```python
from build123d import *

# Parameters (mm, degrees)
SKETCH_1_W          = 60
SKETCH_1_H          = 16
EXTRUDE_1_DEPTH     = 3
SKETCH_2_W          = 60
SKETCH_2_H          = 4
EXTRUDE_2_DEPTH     = 100
SKETCH_3_W          = 5
SKETCH_3_H          = 3
EXTRUDE_3_DEPTH     = 30
CUT_EXTRUDE_2_DEPTH = 12
FILLET_2_R          = 5
SKETCH_6_W          = 5
SKETCH_6_H          = 16
CUT_EXTRUDE_3_DEPTH = 12


with BuildPart() as part:
    # 草图1 → 凸台-拉伸1 (new body)
    with BuildSketch(Plane.XY):
        with Locations((7.850953206, 0.370883882)):
            Rectangle(SKETCH_1_W, SKETCH_1_H)
    extrude(amount=EXTRUDE_1_DEPTH)

    # 草图2 → 凸台-拉伸2 (add)
    with BuildSketch(Plane.XY.offset(3)):
        with Locations((7.850953206, -0.129116118)):
            Rectangle(SKETCH_2_W, SKETCH_2_H)
    extrude(amount=EXTRUDE_2_DEPTH)

    # 草图3 → 凸台-拉伸3 (add)
    with BuildSketch(Plane.XZ.offset(2.129116118)):
        with Locations((-4.649046794, 101.5)):
            Rectangle(SKETCH_3_W, SKETCH_3_H)
        with Locations((20.350953206, 101.5)):
            Rectangle(SKETCH_3_W, SKETCH_3_H)
    extrude(amount=EXTRUDE_3_DEPTH)

    # 草图4 → 切除-拉伸2 (cut)
    with BuildSketch(Plane.XZ.offset(2.129116118)):
        Polygon((-7.149046794, 103), (-22.149046794, 103), (-22.149046794, 3), (-7.149046794, 3), (-7.149046794, 100), align=None)
        Polygon((-2.149046794, 42.479838541), (-2.149046794, 3), (17.850953206, 3), (17.850953206, 10.460890497), (16.154674687, 13.176543186), align=None)
        Polygon((17.850953206, 71.715630146), (17.850953206, 18.011289252), (0.231428364, 46.219221776), align=None)
        Polygon((15.355477041, 75.140410003), (-2.149046794, 49.810414331), (-2.149046794, 96.816642788), align=None)
        Polygon((22.850953206, 100), (22.850953206, 3), (37.850953206, 3), (37.850953206, 103), (22.850953206, 103), align=None)
        Polygon((17.850953206, 100), (17.850953206, 78.416921986), (0.421656, 100), align=None)
    extrude(amount=-CUT_EXTRUDE_2_DEPTH, mode=Mode.SUBTRACT)

    # 圆角2
    fillet_2_edges = [part.edges().sort_by_distance(p)[0] for p in [
        (17.850953206, -0.129116118, 3),
        (-2.149046794, -0.129116118, 3),
        (22.850953206, -0.129116118, 3),
        (20.350953206, 1.870883882, 3),
        (-4.649046794, 1.870883882, 3),
        (-4.649046794, -2.129116118, 3),
        (20.350953206, -2.129116118, 3),
        (-7.149046794, -0.129116118, 3),
    ]]
    fillet(fillet_2_edges, radius=FILLET_2_R)

    # 草图6 → 切除-拉伸3 (cut)
    with BuildSketch(Plane.XY.offset(3)):
        with Locations((-19.649046794, 0.370883882)):
            Rectangle(SKETCH_6_W, SKETCH_6_H)
        with Locations((35.350953206, 0.370883882)):
            Rectangle(SKETCH_6_W, SKETCH_6_H)
    extrude(amount=-CUT_EXTRUDE_3_DEPTH, mode=Mode.SUBTRACT)


solid = part.part
```
Source: CAD feature listing. Evaluate the final solid. Frame: model axes, mm. A direction names the side the tool comes from. Give positions to 0.01 mm unless a question says otherwise; leave off trailing zeros. Loops run counter-clockwise (first coordinate to the right, second up) from the corner with the lowest first, then second, coordinate; pieces in that order, holes last. Notation, with made-up numbers: M 47,16 L 52,16 A35 ccw 52,51 Z; hole C 3.25,17 d3. An arc over 180 degrees is marked long. Put each result on its own line as item: value.
Q1. Section D-D (x = 21). Return the cut outline in (y, z), and give its area (3 significant figures).
Response values:
outline: M -32.13,100 L -2.13,100 L -2.13,8 A5 cw -7.13,3 L -7.63,3 L -7.63,0 L 8.37,0 L 8.37,3 L 6.87,3 A5 cw 1.87,8 L 1.87,103 L -32.13,103 Z
area: 549 mm²
Q2. Line query: probe 1 along Y at (x, z) = (19.5, 59.5); probe 2 along X at (y, z) = (-2, 66.5); probe 3 along Z at (x, y) = (-6, -15.5). Output: solid intervals per line, ascending. Write a range as [from, to].
Response values:
probe 1: y = [-2.13, 1.87]
probe 2: x = [-7.15, -2.15], [9.38, 14.25], [17.85, 22.85]
probe 3: z = [100, 103]
Q3. Section A-A (y = -26). Return the cut outline in (x, z), and give its area (3 significant figures).
Response values:
outline: M -7.15,100 L -2.15,100 L -2.15,103 L -7.15,103 Z; M 17.85,100 L 22.85,100 L 22.85,103 L 17.85,103 Z
area: 30.0 mm²
Q4. Mould query, pull axis Z, two halves, no side actions, for faces 1 (the flat face through (-17.149, 0, 2)), 2 (the flat face through (-2.4, -11.1, 103)), 3 (the cylindrical face through (15.67, -0.03, 3.87)). Classes: released by +Z, released by -Z, zero draft, split by the parting line, or undercut.
Response values:
face 1: zero draft
face 2: released by +Z
face 3: undercut
Q5. Section B-B (y = 0). Return the cut outline in (x, z), and give its area (3 significant figures).
Response values:
outline: M -17.15,0 L 32.85,0 L 32.85,3 L 27.85,3 A5 cw 22.85,8 L 22.85,103 L -7.15,103 L -7.15,8 A5 cw -12.15,3 L -17.15,3 Z; hole M -2.15,8 A5 ccw 2.85,3 L 12.85,3 A5 ccw 17.85,8 L 17.85,10.46 L -2.15,42.48 Z; hole M -2.15,49.81 L 15.36,75.14 L -2.15,96.82 Z; hole M 0.23,46.22 L 17.85,18.01 L 17.85,71.72 Z; hole M 0.42,100 L 17.85,78.42 L 17.85,100 Z
area: 1,630 mm²
Q6. Section C-C (y = -5.5). Return the cut outline in (x, z), and give its area (3 significant figures).
Response values:
outline: M -17.15,0 L 32.85,0 L 32.85,3 L 27.85,3 A5 cw 26.22,3.27 L 14.48,3.27 A5 cw 12.85,3 L 2.85,3 A5 cw 1.22,3.27 L -10.52,3.27 A5 cw -12.15,3 L -17.15,3 Z; M -7.15,100 L -2.15,100 L -2.15,103 L -7.15,103 Z; M 17.85,100 L 22.85,100 L 22.85,103 L 17.85,103 Z
area: 187 mm²
Q7. Reachability of faces 4 (the flat face through (17.851, -17, 101)), 5 (the flat face through (17.851, 0, 9)), 6 (the flat face through (-5, -17, 100)) from +Z, -Z, +X, -X, +Y, -Y: full face, straight path, thin tool, end or side. Return the list, or none.
Response values:
face 4: +Z, -Y
face 5: +Y, -Y
face 6: +X, -X, -Y
Q8. Pin query (flat end, axial travel): P1, Ø3, axis at y = 0.5, z = 56, coming from the +X side; P2, Ø24, axis at x = 4, z = 39, coming from the -Y side; P3, Ø1.5, axis at y = -3.5, z = 45, coming from the +X side (3 decimals); P4, Ø24, axis at x = 2.5, z = 48.5, coming from the +Y side. Return the tip coordinate at first contact, or that it passes through.
Response values:
P1: stops at x = 22.85
P2: stops at y = -2.13
P3: passes through
P4: stops at y = 1.87
